Read the model definition and answer for the solid it produces. Units are mm, in the model's axes. A direction names the side the tool comes from. Give positions to 0.01 mm unless a question says otherwise; leave off trailing zeros. Loops run counter-clockwise (first coordinate to the right, second up) from the corner with the lowest first, then second, coordinate; pieces in that order, holes last. Notation, with made-up numbers: (19, -8) -> (28, -8) arc R26 ccw to (28, 28) -> close; hole circle Ø10 at (53, -6). An arc over 180 degrees is marked (long way). Write each question's results on one line, items separated by ' | '. Start each with the question number.
Item 1: Section D-D on y = 12.25 is taken. Write down the section's boundary in (x, z).
Item 2: Section A-A on y = 0 is taken. Write down the section's boundary in (x, z).
Item 3: Find the intervals of material crossed by line 1 (X direction, y = 8.5, z = 3); line 2 (Y direction, x = 3.5, z = 9.25); line 3 (X direction, y = 9, z = 1.75), in increasing order.
Item 4: Section C-C on x = -1 is taken. Write down the section's boundary in (y, z).
Item 5: Section B-B on z = 4.75 is taken. Write down the section's boundary in (x, y).
Item 6: Determine the mould class of faces 1 (the flat face through (0, -11, 5)), 2 (the cylindrical face through (16.859, 12.797, 5.07)), 3 (the cylindrical face through (-16.859, -12.797, 5.07)) for opening direction X: +X half, -X half, draft (parallel to the pull), parting line (faces both ways), or undercut.
Item 7: Which of the six approach directions +Z, -Z, +X, -X, +Y, -Y give full straight-line access (tool end or side, diameter ignored) to faces 4 (the flat face through (0, -12, 10)), 5 (the cylindrical face through (14.248, -10.287, 5.07))?
```python
from build123d import *

# Parameters (mm, degrees)
F0_W     = 36
F0_H     = 28
F1_DEPTH = 10
F2_T     = -3
F3_R     = 2.5
F4_R     = 4


with BuildPart() as f1:
    # F0 (on Top) → F1 (new body)
    with BuildSketch(Plane.XY):
        Rectangle(F0_W, F0_H)
    extrude(amount=F1_DEPTH)

    # F2
    f2_openings = [f1.faces().sort_by_distance(p)[0] for p in [
        (0, 0, 10),
        (0, 0, 0),
    ]]
    offset(amount=F2_T, openings=f2_openings)

    # F3
    f3_edges = [f1.edges().sort_by_distance(p)[0] for p in [
        (-15, 11, 5),
        (15, 11, 5),
        (-15, -11, 5),
        (15, -11, 5),
    ]]
    fillet(f3_edges, radius=F3_R)

    # F4
    f4_edges = [f1.edges().sort_by_distance(p)[0] for p in [
        (-18, 14, 5),
        (18, 14, 5),
        (-18, -14, 5),
        (18, -14, 5),
    ]]
    fillet(f4_edges, radius=F4_R)


solid = f1.part
```
Findings:
1) outline: (-17.31, 0) -> (17.31, 0) -> (17.31, 10) -> (-17.31, 10) -> close
2) outline: (-18, 0) -> (-15, 0) -> (-15, 10) -> (-18, 10) -> close; (15, 0) -> (18, 0) -> (18, 10) -> (15, 10) -> close
3) line 1: -18 to -15, 15 to 18 | line 2: -14 to -11, 11 to 14 | line 3: -18 to -14.95, 14.95 to 18
4) outline: (-14, 0) -> (-11, 0) -> (-11, 10) -> (-14, 10) -> close; (11, 0) -> (14, 0) -> (14, 10) -> (11, 10) -> close
5) outline: (-18, -10) arc R4 ccw to (-14, -14) -> (14, -14) arc R4 ccw to (18, -10) -> (18, 10) arc R4 ccw to (14, 14) -> (-14, 14) arc R4 ccw to (-18, 10) -> close; hole (-15, -8.5) arc R2.5 ccw to (-12.5, -11) -> (12.5, -11) arc R2.5 ccw to (15, -8.5) -> (15, 8.5) arc R2.5 ccw to (12.5, 11) -> (-12.5, 11) arc R2.5 ccw to (-15, 8.5) -> close
6) face 1: undercut | face 2: +X half | face 3: -X half
7) face 4: +Z, +X, -X, +Y, -Y | face 5: +Z, -Z
